```python
from build123d import *

# Parameters (mm, degrees)
BOSS_EXTRUDE1_START = -2
SKETCH1_R           = 2.5
BOSS_EXTRUDE1_DEPTH = 5.5
BOSS_EXTRUDE2_REACH = 96.191
SKETCH2_R           = 5.5
SKETCH2_R_2         = 2.5
FILLET1_R           = 1.5
FILLET2_R           = 0.5
CHAMFER1_SIZE       = 0.4


with BuildPart() as part:
    # Sketch1 → Boss-Extrude1 (new body)
    with BuildSketch(Plane(origin=(0, -76.733621845, 0), x_dir=(1, 0, 0), z_dir=(0, 1, 0)).offset(BOSS_EXTRUDE1_START)):
        with BuildLine():
            Line((53.041217068, 9.5), (70.045503657, 9.5))
            ThreePointArc((70.045503657, 9.5), (72.332982212, 8.946059138), (74.11360963, 7.406976744))
            Line((74.11360963, 7.406976744), (76.446988808, 4.141579527))
            ThreePointArc((76.446988808, 4.141579527), (82.114772389, 0.763045112), (88.441217068, 2.637708614))
            ThreePointArc((88.441217068, 2.637708614), (90.354455743, 4.667684765), (91.758842367, 7.07786808))
            Line((91.758842367, 7.07786808), (90.378524492, 7.07786808))
            ThreePointArc((90.378524492, 7.07786808), (90.053291089, 6.475468544), (89.691215146, 5.89446684))
            Line((89.691215146, 5.89446684), (88.441217068, 5.89446684))
            Line((88.441217068, 5.89446684), (88.441217068, 12))
            Line((88.441217068, 12), (88.441217068, 13.810660172))
            ThreePointArc((88.441217068, 13.810660172), (86.657690725, 18.116473657), (82.35187724, 19.9))
            Line((82.35187724, 19.9), (80.541217068, 19.9))
            ThreePointArc((80.541217068, 19.9), (76.927000951, 19.024773438), (74.11360963, 16.593023256))
            ThreePointArc((74.11360963, 16.593023256), (72.332982212, 15.053940862), (70.045503657, 14.5))
            Line((70.045503657, 14.5), (53.041217068, 14.5))
            ThreePointArc((53.041217068, 14.5), (50.541217068, 12), (53.041217068, 9.5))
        make_face()
        with Locations(Location((80.541217068, 12, 0), (0, 0, 270))):
            Circle(SKETCH1_R, mode=Mode.SUBTRACT)
    extrude(amount=-BOSS_EXTRUDE1_DEPTH)

    # Sketch2 → Boss-Extrude2 (add, up to next)
    with BuildSketch(Plane(origin=(0, -76.733621845, 0), x_dir=(-1, 0, 0), z_dir=(0, -1, 0)), mode=Mode.PRIVATE) as boss_extrude2_sk1:
        with Locations(Location((-80.541217068, 12, 0), (0, 0, 270))):
            Circle(SKETCH2_R)
        with Locations(Location((-80.541217068, 12, 0), (0, 0, 270))):
            Circle(SKETCH2_R_2, mode=Mode.SUBTRACT)
    boss_extrude2_tool1 = extrude(boss_extrude2_sk1.sketch, amount=BOSS_EXTRUDE2_REACH, mode=Mode.PRIVATE) - part.part
    add(boss_extrude2_tool1.solids().sort_by_distance((80.541217, -76.733622, -17.344437))[0])

    # Fillet1
    fillet1_edges = [part.edges().sort_by_distance(p)[0] for p in [
        (80.541217068, -78.733621845, -17.5),
    ]]
    fillet(fillet1_edges, radius=FILLET1_R)

    # Fillet2
    fillet2_edges = [part.edges().sort_by_distance(p)[0] for p in [
        (89.066216107, -78.733621845, -5.89446684),
        (90.053291089, -78.733621845, -6.475468544),
        (90.354455743, -78.733621845, -4.667684765),
        (82.114772389, -78.733621845, -0.763045112),
        (75.280299219, -78.733621845, -5.774278136),
        (72.332982212, -78.733621845, -8.946059138),
        (61.543360362, -78.733621845, -9.5),
        (50.541217068, -78.733621845, -12),
        (61.543360362, -78.733621845, -14.5),
        (72.332982212, -78.733621845, -15.053940862),
        (76.927000951, -78.733621845, -19.024773438),
        (81.446547154, -78.733621845, -19.9),
        (86.657690725, -78.733621845, -18.116473657),
        (88.441217068, -78.733621845, -9.852563506),
        (88.441217068, -81.483621845, -5.89446684),
        (89.691215146, -81.483621845, -5.89446684),
        (90.378524492, -81.483621845, -7.07786808),
        (91.758842367, -81.483621845, -7.07786808),
        (80.541217068, -76.733621845, -17.5),
    ]]
    fillet(fillet2_edges, radius=FILLET2_R - 0.0001)  # a hair under: the kernel refuses the full size

    # Chamfer1
    chamfer1_edges = [part.edges().sort_by_distance(p)[0] for p in [
        (86.657690725, -84.233621845, -18.116473657),
        (81.446547154, -84.233621845, -19.9),
        (76.927000951, -84.233621845, -19.024773438),
        (72.332982212, -84.233621845, -15.053940862),
        (61.543360362, -84.233621845, -14.5),
        (50.541217068, -84.233621845, -12),
        (61.543360362, -84.233621845, -9.5),
        (80.541217068, -84.233621845, -14.5),
        (72.332982212, -84.233621845, -8.946059138),
        (75.280299219, -84.233621845, -5.774278136),
        (82.114772389, -84.233621845, -0.763045112),
        (90.106673865, -84.233621845, -4.347253026),
        (90.0483511, -84.233621845, -6.46697167),
        (90.824107859, -84.233621845, -7.07786808),
        (89.180451269, -84.233621845, -5.89446684),
        (88.441217068, -84.233621845, -10.102513506),
        (90.425701502, -84.233621845, -7.006759492),
        (91.39286189, -84.233621845, -6.837375819),
        (89.661122586, -84.233621845, -5.95658104),
        (88.587634388, -84.233621845, -6.04088416),
    ]]
    chamfer(chamfer1_edges, length=CHAMFER1_SIZE)


solid = part.part
```
CAD build for the part. Positions are in the model's coordinates, mm. A direction names the side the tool comes from. Coordinates: 2 decimals unless noted, no trailing zeros. Order: outer loops, then holes, each group sorted by start corner. A loop starts at its lowest first (then second) coordinate and runs counter-clockwise, first axis right, second up. Notation, with made-up numbers: (-14.75, 85.25) - (-8.75, 85.25) arc R14 cw to (-8.75, 91.25) - close; hole circle Ø3 at (82.25, 41). An arc over 180 degrees is marked (long way). Answer in a Markdown table with one row per item.
1. Drill centre lines: L1, parallel to X at y = -81.5, z = -12; L2, parallel to Y at x = 88.5, z = -4.75; L3, parallel to Z at x = 54.5, y = -83. Where is each one in solid material? Low to high. Write a range as from..to.
Answer:
| item | result |
|---|---|
| L1 | 50.54..78.04, 83.04..88.44 |
| L2 | -84.23..-78.73 |
| L3 | -14.5..-9.5 |
2. Flat gauge pins, fed straight in: P1, Ø1.4, axis at x = 62, y = -82, coming from the -Z side; P2, Ø6, axis at x = 61, z = -7, coming from the +Y side; P3, Ø2.5, axis at y = -81, z = -9, coming from the +X side; P4, Ø3, axis at x = 80.54, z = -12, coming from the +Y side. Where does each tip first touch, or does it go through?
Answer:
| item | result |
|---|---|
| P1 | z = -14.5 |
| P2 | y = -78.73 |
| P3 | x = 88.44 |
| P4 | through |
3. 3-axis set-ups, long thin cutter, end or side, ignore diameter. For faces 1 (the face through (62, -82, -14.5)), 2 (the face through (88.48, -83.99, -5.93)), 3 (the face through (72.352, -83.942, -9.058)): which of +Z, -Z, +X, -X, +Y, -Y reach the whole face in a straight line?
Answer:
| item | result |
|---|---|
| face 1 | -Z, -X, +Y, -Y |
| face 2 | -Z, -Y |
| face 3 | +Z, -X, -Y |
4. Slice it at B-B, the plane x = 68. List the corners of the cut face in (y, z).
Answer:
| item | result |
|---|---|
| outline | (-84.23, -14.1) - (-83.83, -14.5) - (-79.23, -14.5) arc R0.5 ccw to (-78.73, -14) - (-78.73, -10) arc R0.5 ccw to (-79.23, -9.5) - (-83.83, -9.5) - (-84.23, -9.9) - close |
